from build123d import *

# Parameters (mm, degrees)
SKETCH1_R           = 2.413
SKETCH1_W           = 6.35
SKETCH1_H           = 6.35
BOSS_EXTRUDE1_DEPTH = 6.35


with BuildPart() as part:
    # Sketch1 → Boss-Extrude1 (new body)
    with BuildSketch(Plane(origin=(0, 0, 0), x_dir=(1, 0, 0), z_dir=(0, 1, 0))):
        with BuildLine():
            Line((-4.276232573, 19.216684391), (-37.939187052, 19.216684391))
            ThreePointArc((-37.939187052, 19.216684391), (-41.464378908, 19.715740887), (-44.712520386, 21.17368874))
            Line((-44.712520386, 21.17368874), (-62.328552859, 32.280391547))
            ThreePointArc((-62.328552859, 32.280391547), (-66.67527648, 36.888704376), (-68.255219526, 43.023387198))
            Line((-68.255219526, 43.023387198), (-68.255219526, 57.951684391))
            ThreePointArc((-68.255219526, 57.951684391), (-70.115091465, 62.441812452), (-74.605219526, 64.301684391))
            Line((-74.605219526, 64.301684391), (-103.180219526, 64.301684391))
            ThreePointArc((-103.180219526, 64.301684391), (-108.250679153, 60.73228976), (-111.435219526, 55.411684391))
            ThreePointArc((-111.435219526, 55.411684391), (-119.055219526, 9.691684391), (-111.435219526, -36.028315609))
            ThreePointArc((-111.435219526, -36.028315609), (-108.250679153, -41.348920977), (-103.180219526, -44.918315609))
            Line((-103.180219526, -44.918315609), (-74.605219526, -44.918315609))
            ThreePointArc((-74.605219526, -44.918315609), (-70.115091465, -43.058443669), (-68.255219526, -38.568315609))
            Line((-68.255219526, -38.568315609), (-68.255219526, -23.640018416))
            ThreePointArc((-68.255219526, -23.640018416), (-66.67527648, -17.505335593), (-62.328552859, -12.897022765))
            Line((-62.328552859, -12.897022765), (-44.712520386, -1.790319958))
            ThreePointArc((-44.712520386, -1.790319958), (-41.464378908, -0.332372105), (-37.939187052, 0.166684391))
            Line((-37.939187052, 0.166684391), (-27.387614836, 0.166684391))
            Line((-27.387614836, 0.166684391), (-24.553673229, 0.166684391))
            ThreePointArc((-24.553673229, 0.166684391), (-19.165519557, -2.065161936), (-16.933673229, -7.453315609))
            Line((-16.933673229, -7.453315609), (-11.696120928, -38.563381903))
            ThreePointArc((-11.696120928, -38.563381903), (-9.102466616, -43.116571583), (-4.181867321, -44.918315609))
            Line((-4.181867321, -44.918315609), (-1.580219526, -44.918315609))
            ThreePointArc((-1.580219526, -44.918315609), (3.807934147, -42.686469281), (6.039780474, -37.298315609))
            Line((6.039780474, -37.298315609), (6.039780474, -36.576031258))
            ThreePointArc((6.039780474, -36.576031258), (6.010508622, -36.031471642), (5.923030406, -35.493187723))
            Line((5.923030406, -35.493187723), (2.657517771, -20.525600214))
            ThreePointArc((2.657517771, -20.525600214), (2.220126687, -17.834180618), (2.073767427, -15.111382542))
            Line((2.073767427, -15.111382542), (2.073767427, 5.246684391))
            Line((2.073767427, 5.246684391), (2.073767427, 12.866684391))
            ThreePointArc((2.073767427, 12.866684391), (0.213895488, 17.356812452), (-4.276232573, 19.216684391))
        make_face()
        with Locations((-103.180219526, -36.028315609)):
            Circle(SKETCH1_R, mode=Mode.SUBTRACT)
        with Locations((-77.780219526, -36.028315609)):
            Circle(SKETCH1_R, mode=Mode.SUBTRACT)
        with Locations((-77.780219526, -23.328315609)):
            Circle(SKETCH1_R, mode=Mode.SUBTRACT)
        with Locations((-77.780219526, -10.628315609)):
            Rectangle(SKETCH1_W, SKETCH1_H, mode=Mode.SUBTRACT)
        with Locations((-1.580219526, -36.028315609)):
            Circle(SKETCH1_R, mode=Mode.SUBTRACT)
        with Locations((-7.451232573, -7.453315609)):
            Circle(SKETCH1_R, mode=Mode.SUBTRACT)
        with Locations((-111.435219526, 9.691684391)):
            Circle(SKETCH1_R, mode=Mode.SUBTRACT)
        with Locations((-77.780219526, 30.011684391)):
            Rectangle(SKETCH1_W, SKETCH1_H, mode=Mode.SUBTRACT)
        with Locations((-103.180219526, 55.411684391)):
            Circle(SKETCH1_R, mode=Mode.SUBTRACT)
        with Locations((-77.780219526, 42.711684391)):
            Circle(SKETCH1_R, mode=Mode.SUBTRACT)
        with Locations((-77.780219526, 55.411684391)):
            Circle(SKETCH1_R, mode=Mode.SUBTRACT)
        with Locations((-45.551232573, 9.691684391)):
            Rectangle(SKETCH1_W, SKETCH1_H, mode=Mode.SUBTRACT)
        with Locations((-7.451232573, 9.691684391)):
            Rectangle(SKETCH1_W, SKETCH1_H, mode=Mode.SUBTRACT)
    extrude(amount=BOSS_EXTRUDE1_DEPTH)


solid = part.part
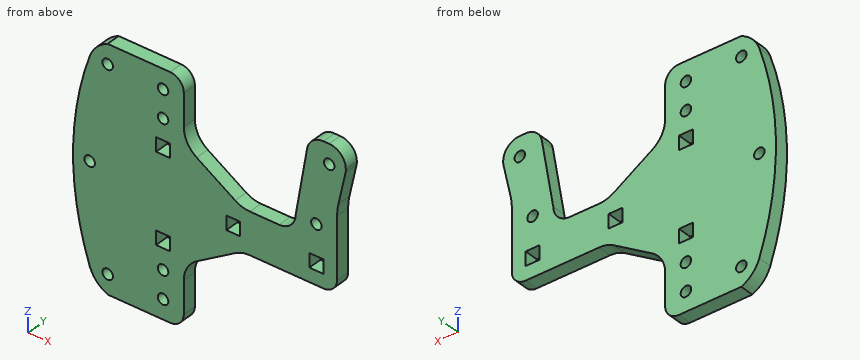
Design review of the part built by this model. Coordinates are the model's own, in mm. Give positions to 0.01 mm unless a question says otherwise; leave off trailing zeros. Loops run counter-clockwise (first coordinate to the right, second up) from the corner with the lowest first, then second, coordinate; pieces in that order, holes last. Notation, with made-up numbers: M 63.5,7.5 L 67.5,7.5 A22 cw 67.5,21.5 Z; hole C 69.5,7.5 d9. An arc over 180 degrees is marked long. Write item = value, one per line.
Q1. We need section C-C (y = 1.5). Count the separate pieces of the cut face and the enclosed holes in it, plus the area to 3 significant figures.
Output values:
separate_pieces = 1
enclosed_holes = 13
area = 7,390 mm^2
Q2. We need section B-B (x = -27.5). Give the boundary of the cut face in (y, z), plus the area to 3 significant figures.
Output values:
outline = M 0,-19.22 L 6.35,-19.22 L 6.35,-0.17 L 0,-0.17 Z
area = 121 mm^2
Q3. To check wall thickness, follow line 1 (X direction, y = 3, z = -10); line 2 (Z direction, x = -5.5, y = 2); line 3 (X direction, y = 5.25, z = 24). State the ranges of each line that lie inside material, in increasing order. Write a range as [from, to].
Output values:
line_1 = [-119.05, -113.83], [-109.04, -48.73], [-42.38, -10.63], [-4.28, 2.07]
line_2 = [-19.22, -12.87], [-6.52, 6.03], [8.87, 44.8]
line_3 = [-114.97, -80.1], [-75.46, -68.26], [-14.15, 3.42]
Q4. We need section A-A (z = 28). Give the boundary of the cut face in (x, y), plus the area to 3 significant figures.
Output values:
outline = M -113.92,0 L -68.26,0 L -68.26,6.35 L -113.92,6.35 Z; M -13.47,0 L 4.29,0 L 4.29,6.35 L -13.47,6.35 Z
area = 403 mm^2
Q5. We need section D-D (z = -48.5). Give the boundary of the cut face in (x, y), plus the area to 3 significant figures.
Output values:
outline = M -113.61,0 L -68.26,0 L -68.26,6.35 L -113.61,6.35 Z
area = 288 mm^2
Q6. Insertion check: pin 1 (3 mm diameter, centred on x = -77.78, z = -42.71, fed in from +Y); pin 2 (1.5 mm diameter, centred on x = -51.5, y = 1.5, fed in from +Z); pin 3 (1 mm diameter, centred on y = 4.5, z = 28, fed in from -X); pin 4 (3 mm diameter, centred on x = -26, y = 3.5, fed in from -Z). Each pin has a flat end and moves straight along its axis. Give the tip position at first contact, or say it passes through.
Output values:
pin_1 = through
pin_2 = 6.54
pin_3 = -114.06
pin_4 = -19.22
